The figure shows three views and two pictorial views of one solid part (mm, origin at its lowest corner). Answer the questions. A direction names the side the tool comes from. Give positions to 0.01 mm unless a question says otherwise; leave off trailing zeros. Write each loop counter-clockwise with the first axis right and the second up, starting at its lowest first coordinate (ties: lowest second). Pieces come first, ordered by that corner, then holes. Notation, with made-up numbers: (74, 50.5) - (87, 50.5) arc R21 cw to (87, 81.5) - close; hole circle Ø7 at (30.5, 34.25). An arc over 180 degrees is marked (long way). Answer as CSV lines item,"result". Start each with the question number.
(1) Find section C-C (y = 7.5). Write down the section's boundary in (x, z), then the cut area to 3 significant figures.
(2) Find section A-A (x = 15.75). Write down the section's boundary in (y, z) (3 decimals), then the cut area to 4 significant figures.
(3) For the marked faces 5, 6 and 7, determine the directions among +Z, -Z, +X, -X, +Y, -Y from which every point of the face is accessible in a straight line to the end or side of a thin tool.
(4) For a pull along Y with two mould halves and no side action, classify the marked faces 1, 2, 3 and 4 as pulls with the +Y half, pulls with the -Y half, needs draft (parallel to the pull), parting line crosses it, or undercut.
(5) Find section B-B (z = 1.8). State how many separate pieces and enclosed holes the cut face has, then the cut area to 3 significant figures.
(6) Each of these flat-tipped pins is pushed along its axis until it touches: pin 1 Ø0.9 at (y, z) = (7, 2) entering from -X; pin 2 Ø1.5 at (x, y) = (4, 11.5) entering from -Z; pin 3 Ø2 at (x, y) = (13, 3.5) entering from -Z; pin 4 Ø0.9 at (x, z) = (5, 1.5) entering from -Y. Where does it stop, or does it pass through?
(7) Straight lines are drawn through the part: probe 1 along X at (y, z) = (13.5, 1.2); probe 2 along Y at (x, z) = (16, 1.25) (3 decimals); probe 3 along Y at (x, z) = (14, 0.95) (3 decimals). For each, find the intervals that lie inside material, in ascending order.
(8) Find section D-D (y = 10). Write down the section's boundary in (x, z), then the cut area to 3 significant figures.
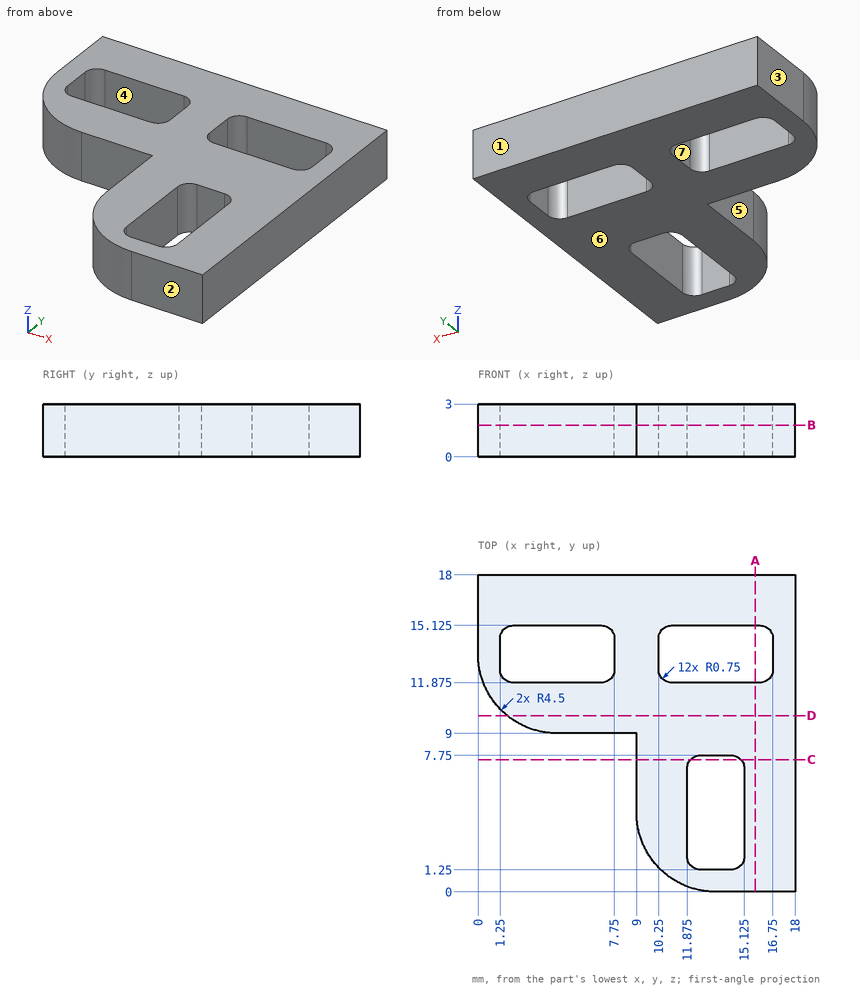
Result set:
1,outline,"(9, 0) - (12.07, 0) - (12.07, 3) - (9, 3) - close; (14.93, 0) - (18, 0) - (18, 3) - (14.93, 3) - close"
1,area,"18.4 mm^2"
2,outline,"(0, 0) - (11.875, 0) - (11.875, 3) - (0, 3) - close; (15.125, 0) - (18, 0) - (18, 3) - (15.125, 3) - close"
2,area,"44.25 mm^2"
3,face 5,"+Z, -Z, -X, -Y"
3,face 6,"-Z, +X, -X, +Y, -Y"
3,face 7,"+Z, -Z"
4,face 1,"pulls with the +Y half"
4,face 2,"pulls with the -Y half"
4,face 3,"needs draft"
4,face 4,"undercut"
5,separate pieces,"1"
5,enclosed holes,"3"
5,area,"172 mm^2"
6,pin 1,"x = 9"
6,pin 2,"z = 0"
6,pin 3,"through"
6,pin 4,"y = 9"
7,probe 1,"0 to 1.25, 7.75 to 10.25, 16.75 to 18"
7,probe 2,"0 to 11.875, 15.125 to 18"
7,probe 3,"0 to 1.25, 7.75 to 11.875, 15.125 to 18"
8,outline,"(1.67, 0) - (18, 0) - (18, 3) - (1.67, 3) - close"
8,area,"49.0 mm^2"
